Build history of the part. All positions in model axes, mm. Round coordinates to 2 decimals unless told otherwise and drop trailing zeros. Write each loop counter-clockwise with the first axis right and the second up, starting at its lowest first coordinate (ties: lowest second). Pieces come first, ordered by that corner, then holes. Notation, with made-up numbers: M 45,44 L 54,44 A36 cw 54,79 Z; hole C 13,-35 d9. An arc over 180 degrees is marked long. Write item = value, one per line.
Autodesk Inventor part; units mm, degrees
ref_plane "YZ Plane" through (0, 0, 0) normal (1, 0, 0) x (0, 1, 0)
ref_plane "XZ Plane" through (0, 0, 0) normal (0, 1, 0) x (-1, 0, 0)
ref_plane "XY Plane" through (0, 0, 0) normal (0, 0, 1) x (1, 0, 0)
sketch "スケッチ1" plane through (0, 0, 0) normal (0, 0, 1) x (1, 0, 0)
  line L0 (-40, 12) -> (40, 12)
  line L1 (40, 12) -> (40, -12)
  line L2 (40, -12) -> (-40, -12)
  line L3 (-40, -12) -> (-40, 12)
  point P0 (0, 0)
  dimension "d0" = 80
  dimension "d1" = 24
  dimension "d2" = 12
  dimension "d3" = 40
extrude "押し出し1" add sketch "スケッチ1" along normal blind 5
sketch "スケッチ2" plane through (0, 0, 5) normal (0, 0, 1) x (1, 0, 0)
  line L0 (-0.8, 9.8) -> (35, 9.8)
  line L1 (35, 9.8) -> (35, -9.8)
  line L2 (35, -9.8) -> (-0.8, -9.8)
  line L3 (-0.8, -9.8) -> (-0.8, 9.8)
  line L4 (35, 9.8) -> (30.75, 9.8)
  line L5 (30.75, 9.8) -> (30.75, -9.8)
  line L6 (30.75, -9.8) -> (35, -9.8)
  line L7 (35, -9.8) -> (35, 9.8)
  line L8 (30.75, -9.8) -> (14.75, -9.8)
  line L9 (14.75, -9.8) -> (14.75, 9.8)
  line L10 (14.75, 9.8) -> (30.75, 9.8)
  line L11 (30.75, 9.8) -> (30.75, -9.8)
  circle A0 centre (8, 0) radius 5
  line L12 (35, 0) -> (-0.8, 0)
  circle A1 centre (1.8, 7.2) radius 1.25
  circle A2 centre (32.9, 7.7) radius 1.25
  circle A3 centre (1.8, -7.2) radius 1.25
  circle A4 centre (32.9, -7.7) radius 1.25
  line L13 (40, 12) -> (40, -12)
  point P0 (0, 0)
  dimension "d6" = 35.8
  dimension "d7" = 19.6
  dimension "d8" = 9.8
  dimension "d10" = 4.25
  dimension "d11" = 16
  dimension "d12" = 10
  dimension "d13" = 27
  dimension "d14" = 14.4
  dimension "d15" = 15.4
  dimension "d16" = 31.1
  dimension "d17" = 2.1
  dimension "d18" = 2.5
  dimension "d19" = 2.5
  dimension "d47" = 5
extrude "押し出し2" cut sketch "スケッチ2" against normal through all contours L0 L5 L12 L9 | L12 L5 L2 L9 | L12 A0 | A0 L12 | A1 | A2 | A3 | A4
fillet "フィレット1" radius 5 2 edges at (14.75, 9.8, 2.5) (14.75, -9.8, 2.5)
fillet "フィレット2" radius 1 2 edges at (30.75, 9.8, 2.5) (30.75, -9.8, 2.5)
sketch "スケッチ5" plane through (0, 0, 5) normal (0, 0, 1) x (1, 0, 0)
  line L0 (40, 12) -> (40, -12)
  line L1 (29.75, -9.8) -> (19.75, -9.8)
  arc A0 (14.75, -4.8) -> (19.75, -9.8) centre (19.75, -4.8) ccw
  line L2 (14.75, -4.8) -> (14.75, 4.8)
  arc A1 (19.75, 9.8) -> (14.75, 4.8) centre (19.75, 4.8) ccw
  line L3 (19.75, 9.8) -> (29.75, 9.8)
  arc A2 (30.75, 8.8) -> (29.75, 9.8) centre (29.75, 8.8) ccw
  line L4 (30.75, 8.8) -> (30.75, -8.8)
  arc A3 (29.75, -9.8) -> (30.75, -8.8) centre (29.75, -8.8) ccw
  circle A4 centre (32.9, -7.7) radius 1.25
  circle A5 centre (1.8, -7.2) radius 1.25
  circle A6 centre (32.9, 7.7) radius 1.25
  circle A7 centre (1.8, 7.2) radius 1.25
  circle A8 centre (8, 0) radius 5
  line L5 (40, 10) -> (-40, 10)
  line L6 (-40, 10) -> (-40, -10)
  line L7 (-40, -10) -> (40, -10)
  line L8 (40, -10) -> (40, 10)
  point P0 (-32.5, 14.4762)
  point P1 (-32.5, -14.4762)
  point P2 (0, 0)
  dimension "d41" = 20
  dimension "d42" = 10
  dimension "d49" = 41.8
extrude "押し出し4" cut sketch "スケッチ5" against normal blind 3
fillet "フィレット3" radius 12 4 edges at (40, -12, 2.5) (40, 12, 2.5) (-40, -12, 2.5) (-40, 12, 2.5)
fillet "フィレット4" radius 0.5 4 edges at (-34.6333, -10, 3.5) (-34.6333, 10, 3.5) (34.6333, 10, 3.5) (34.6333, -10, 3.5)
sketch "スケッチ6" plane through (0, 0, 2) normal (0, 0, 1) x (1, 0, 0)
  circle A0 centre (32.9, -7.7) radius 1.25
  circle A1 centre (26.72, 0) radius 6.5
  point P0 (0, 0)
  dimension "d52" = 13
  dimension "d53" = 6.18
extrude "押し出し5" cut sketch "スケッチ6" against normal through all contours A1
sketch "スケッチ7" plane through (0, 0, 2) normal (0, 0, 1) x (1, 0, 0)
  circle A0 centre (1.8, -7.2) radius 1.25
  circle A1 centre (1.8, 7.2) radius 1.25
  point P0 (0, 0)
  point P1 (-6.2, 7.2)
  point P2 (-6.2, -7.2)
  point P3 (-21.2, -7.2)
  point P4 (-21.2, 7.2)
  point P5 (-6.2, 7.2)
  point P6 (-21.2, 7.2)
  dimension "d56" = 15
  dimension "d57" = 15
  dimension "d58" = 8
  dimension "d59" = 8
  dimension "d60" = 7.2
  dimension "d61" = 7.2
  dimension "d62" = 7.2
  dimension "d63" = 7.2
hole "Hole2" at (-6.2, 7.2, 2) at (-6.2, -7.2, 2) at (-21.2, -7.2, 2) at (-21.2, 7.2, 2) direction (0, 0, -1) diameter 2.5 end through all
properties part number "JointD0"
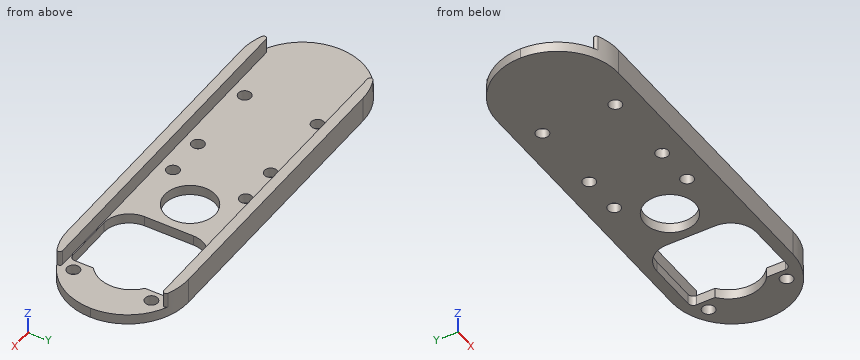
1. Probe probe 1 along Y at (x, z) = (-25.5, 2.4); probe 2 along Y at (x, z) = (1.8, 0.4); probe 3 along X at (y, z) = (-1, 1.6). List the from-to ranges inside material, lowest first.
Responses:
probe_1 = -12 to -10, 10 to 12
probe_2 = -12 to -8.45, -5.95 to 5.95, 8.45 to 12
probe_3 = -39.96 to 3.1, 12.9 to 14.75, 33.14 to 39.96
2. Band-saw the part on A-A (x = 8). List the corners of the cut face in (y, z), plus the area to 3 significant figures.
Responses:
outline = M -12,0 L -5,0 L -5,2 L -10,2 L -10,5 L -12,5 Z; M 5,0 L 12,0 L 12,5 L 10,5 L 10,2 L 5,2 Z
area = 40.0 mm²
3. Band-saw the part on B-B (x = -21.2). List the corners of the cut face in (y, z), plus the area to 3 significant figures.
Responses:
outline = M -12,0 L -8.45,0 L -8.45,2 L -10,2 L -10,5 L -12,5 Z; M -5.95,0 L 5.95,0 L 5.95,2 L -5.95,2 Z; M 8.45,0 L 12,0 L 12,5 L 10,5 L 10,2 L 8.45,2 Z
area = 50.0 mm²
4. Band-saw the part on D-D (z = 4.1). List the corners of the cut face in (x, y), plus the area to 3 significant figures.
Responses:
outline = M -32.89,-10.96 A12 ccw -28,-12 L 28,-12 A12 ccw 32.89,-10.96 A0.5 ccw 32.69,-10 L -32.69,-10 A0.5 ccw Z; M -32.89,10.96 A0.5 ccw -32.69,10 L 32.69,10 A0.5 ccw 32.89,10.96 A12 ccw 28,12 L -28,12 A12 ccw Z
area = 257 mm²
5. Band-saw the part on C-C (x = -9.5). List the corners of the cut face in (y, z).
Responses:
outline = M -12,0 L 12,0 L 12,5 L 10,5 L 10,2 L -10,2 L -10,5 L -12,5 Z
6. Flat gauge pins, fed straight in: pin 1 (1 mm diameter, centred on y = -2, z = 1, fed in from +X); pin 2 (1.6 mm diameter, centred on y = -7, z = 1, fed in from -X); pin 3 (4 mm diameter, centred on x = 1.8, y = 7.2, fed in from +Z). Where does each tip first touch, or does it go through?
Responses:
pin_1 = 39.91
pin_2 = -38.27
pin_3 = 2
